Source: CAD feature listing. Evaluate the final solid. Frame: model axes, mm. A direction names the side the tool comes from. Give positions to 0.01 mm unless a question says otherwise; leave off trailing zeros. Loops run counter-clockwise (first coordinate to the right, second up) from the corner with the lowest first, then second, coordinate; pieces in that order, holes last. Notation, with made-up numbers: M 29,8.5 L 74,8.5 A27 cw 74,26.5 Z; hole C 74.25,73 d10. An arc over 180 degrees is marked long. Put each result on its own line as item: value.
from build123d import *

# Parameters (mm, degrees)
BOSS_EXTRUDE1_DEPTH = 5.18
CUT_EXTRUDE1_REACH  = 36.536
SKETCH2_W           = 3.45
SKETCH2_H           = 5.15
SKETCH3_W           = 10.5
SKETCH3_H           = 30
SKETCH3_R           = 1.575
BOSS_EXTRUDE2_DEPTH = 1.5
CUT_EXTRUDE3_REACH  = 43.242
SKETCH7_R           = 1.575


with BuildPart() as part:
    # Sketch1 → Boss-Extrude1 (new body)
    with BuildSketch(Plane(origin=(0, 0, 0), x_dir=(0, 0, -1), z_dir=(1, 0, 0))):
        Polygon((0, 0), (13, 0), (13, -7.5), (8.2, -7.5), (8.2, -11.6), (13.8, -11.6), (13.8, -10.716666667), (9.8, -10.716666667), (9.8, -10.9), (8.7, -10.9), (8.7, -8), (9.8, -8), (9.8, -8.183333333), (11.3, -8.183333333), (11.3, -8), (14.1, -8), (14.1, -8.183333333), (15.6, -8.183333333), (15.6, -8), (16.7, -8), (16.7, -9.1), (16.516666667, -9.1), (16.516666667, -11.1), (16.7, -11.1), (16.7, -16.35), (16.516666667, -16.35), (16.516666667, -18.35), (17.583333333, -18.35), (17.583333333, -16.35), (17.4, -16.35), (17.4, -11.1), (17.583333333, -11.1), (17.583333333, -9.1), (17.4, -9.1), (17.4, -8), (20.3, -8), (21.8, -19.95), (21.8, -21.45), (0, -21.45), (0, -24.78), (3, -24.78), (3, -26.28), (-1.5, -26.28), (-1.5, -19.95), (0, -8), (2.9, -8), (2.9, -9.5), (2.716666667, -9.5), (2.716666667, -11.5), (2.9, -11.5), (2.9, -16.15), (2.716666667, -16.15), (2.716666667, -18.15), (2.9, -18.15), (2.9, -18.333333333), (4.4, -18.333333333), (4.4, -18.15), (7.2, -18.15), (7.2, -18.333333333), (8.7, -18.333333333), (8.7, -17.266666667), (4.7, -17.266666667), (4.7, -17.45), (3.6, -17.45), (3.6, -7.5), (0, -7.5), align=None)
        Polygon((14.9, -9.8), (14.9, -15.65), (4.7, -15.65), (4.7, -16.533333333), (8.7, -16.533333333), (8.7, -16.35), (9.8, -16.35), (9.8, -19.25), (8.7, -19.25), (8.7, -19.066666667), (7.2, -19.066666667), (7.2, -19.25), (4.4, -19.25), (4.4, -19.066666667), (2.9, -19.066666667), (2.9, -19.25), (1.8, -19.25), (1.8, -18.15), (1.983333333, -18.15), (1.983333333, -16.15), (1.8, -16.15), (1.8, -11.5), (1.983333333, -11.5), (1.983333333, -9.5), (1.1, -9.5), (1.1, -19.95), (19.2, -19.95), (19.2, -9.1), (18.316666667, -9.1), (18.316666667, -11.1), (18.5, -11.1), (18.5, -16.35), (18.316666667, -16.35), (18.316666667, -18.35), (18.5, -18.35), (18.5, -19.45), (15.6, -19.45), (15.6, -18.35), (15.783333333, -18.35), (15.783333333, -16.35), (15.6, -16.35), (15.6, -11.1), (15.783333333, -11.1), (15.783333333, -9.1), (15.6, -9.1), (15.6, -8.916666667), (14.1, -8.916666667), (14.1, -9.1), (11.3, -9.1), (11.3, -8.916666667), (9.8, -8.916666667), (9.8, -9.983333333), (13.8, -9.983333333), (13.8, -9.8), align=None, mode=Mode.SUBTRACT)
    extrude(amount=BOSS_EXTRUDE1_DEPTH)

    # Sketch2 → Cut-Extrude1 (cut, up to next)
    with BuildSketch(Plane.XY, mode=Mode.PRIVATE) as cut_extrude1_sk1:
        with Locations((3.455, -3.425)):
            Rectangle(SKETCH2_W, SKETCH2_H)
    cut_extrude1_tool1 = extrude(cut_extrude1_sk1.sketch, amount=-CUT_EXTRUDE1_REACH, mode=Mode.PRIVATE) & part.part
    add(cut_extrude1_tool1.solids().sort_by_distance((3.455, -3.425, 0))[0], mode=Mode.SUBTRACT)

    # Sketch3 → Boss-Extrude2 (add)
    with BuildSketch(Plane.XZ.offset(21.45)):
        with Locations((5.25, -15)):
            Rectangle(SKETCH3_W, SKETCH3_H)
        with Locations(Location((7.62, -14.98, 0), (0, 0, 270))):
            Circle(SKETCH3_R, mode=Mode.SUBTRACT)
        with Locations(Location((7.62, -26.98, 0), (0, 0, 270))):
            Circle(SKETCH3_R, mode=Mode.SUBTRACT)
    extrude(amount=-BOSS_EXTRUDE2_DEPTH)

    # Sketch7 → Cut-Extrude3 (cut, up to next)
    with BuildSketch(Plane.ZY, mode=Mode.PRIVATE) as cut_extrude3_sk1:
        with Locations((-3.25, -3.5)):
            Circle(SKETCH7_R)
    cut_extrude3_tool1 = extrude(cut_extrude3_sk1.sketch, amount=-CUT_EXTRUDE3_REACH, mode=Mode.PRIVATE) & part.part
    # Sketch7 → Cut-Extrude3 (cut, up to next)
    with BuildSketch(Plane.ZY, mode=Mode.PRIVATE) as cut_extrude3_sk2:
        with Locations((-9.75, -3.5)):
            Circle(SKETCH7_R)
    cut_extrude3_tool2 = extrude(cut_extrude3_sk2.sketch, amount=-CUT_EXTRUDE3_REACH, mode=Mode.PRIVATE) & part.part
    add(cut_extrude3_tool1.solids().sort_by_distance((0, -3.5, -3.25))[0], mode=Mode.SUBTRACT)
    add(cut_extrude3_tool2.solids().sort_by_distance((0, -3.5, -9.75))[0], mode=Mode.SUBTRACT)


with BuildPart() as body_2:
    # Mirror3: mirrored copy
    add(part.part.mirror(Plane(origin=(0, 0, 0), x_dir=(0, 0, 1), z_dir=(1, 0, 0))))


solid = body_2.part
1. Section query B-B (x = -7.62). Output: boundary loops of the cut face in (y, z) (3 decimals), plus the area to 4 significant figures.
Found:
outline: M -21.45,-30 L -19.95,-30 L -19.95,-28.555 L -21.45,-28.555 Z; M -21.45,-25.405 L -19.95,-25.405 L -19.95,-16.555 L -21.45,-16.555 Z; M -21.45,-13.405 L -19.95,-13.405 L -19.95,0 L -21.45,0 Z
area: 35.55 mm^2
2. Access query for faces 4 (the flat face through (-3, -26.28, -1)), 5 (the flat face through (-3, -7.5, -2)), 6 (the flat face through (-3, -26, -3)), 7 (the flat face through (-3, -14, -18.5)). Directions: +Z, -Z, +X, -X, +Y, -Y. A direction counts if a zero-diameter tool reaches every point of the face in a straight line with its end or side. Return the directions, or none.
Found:
face 4: +Z, -Z, +X, -X, -Y
face 5: +Z, +X, -X
face 6: -Z, +X, -X, -Y
face 7: +X, -X
3. Material intervals for line 1 (Z direction, x = -7.62, y = -20.5) (3 decimals); line 2 (Y direction, x = -1.2, z = -3.25) (3 decimals); line 3 (Z direction, x = -2.75, y = -9.25), sorted ascending. Write a range as from..to.
Found:
line 1: -30..-28.555, -25.405..-16.555, -13.405..0
line 2: -21.45..-19.95, -19.067..-18.333, -7.5..-5.075, -1.925..0
line 3: -20.46..-19.2, -18.32..-17.58, -16.52..-15.78, -9.8..-8.7, -8.2..-3.6, -2.9..0.16
4. Section query A-A (y = -3.5). Output: boundary loops of the cut face in (x, z) (3 decimals), plus the area to 3 significant figures.
Found:
outline: M -1.73,-13 L 0,-13 L 0,-11.325 L -1.73,-11.325 Z; M -1.73,-8.175 L 0,-8.175 L 0,-4.825 L -1.73,-4.825 Z; M -1.73,-1.675 L 0,-1.675 L 0,0 L -1.73,0 Z
area: 11.6 mm^2
5. Section query D-D (y = -14). Output: boundary loops of the cut face in (x, z).
Found:
outline: M -5.18,-21.05 L 0,-21.05 L 0,-19.2 L -5.18,-19.2 Z; M -5.18,-18.5 L 0,-18.5 L 0,-17.4 L -5.18,-17.4 Z; M -5.18,-16.7 L 0,-16.7 L 0,-15.6 L -5.18,-15.6 Z; M -5.18,-14.9 L 0,-14.9 L 0,-3.6 L -5.18,-3.6 Z; M -5.18,-2.9 L 0,-2.9 L 0,-1.8 L -5.18,-1.8 Z; M -5.18,-1.1 L 0,-1.1 L 0,0.75 L -5.18,0.75 Z
6. Draft query along Y for faces 1 (the flat face through (-3, -17, -17.583)), 2 (the flat face through (-5, -21, -30)), 3 (the flat face through (-3, 0, -6)). Return one class per face: pulls with the +Y half, pulls with the -Y half, needs draft (parallel to the pull), parting line crosses it, or undercut.
Found:
face 1: undercut
face 2: needs draft
face 3: pulls with the +Y half
7. Contact query for flat-ended pins moving along their axis: P1, Ø1, axis at y = -22, z = -8.5, coming from the +X side; P2, Ø5.5, axis at x = -1.5, y = -14.5, coming from the +Z side; P3, Ø5.5, axis at x = -2.5, y = -3, coming from the +Z side; P4, Ø1, axis at x = -1.5, y = -17.5, coming from the -Z side. Output: stop coordinate, or through.
Found:
P1: through
P2: z = 1.16
P3: z = 0
P4: z = -21.56
8. Section query C-C (z = -4). Output: boundary loops of the cut face in (x, y).
Found:
outline: M -10.5,-21.45 L 0,-21.45 L 0,-19.95 L -10.5,-19.95 Z; M -5.18,-19.07 L 0,-19.07 L 0,-18.33 L -5.18,-18.33 Z; M -5.18,-17.45 L 0,-17.45 L 0,-4.88 L -1.73,-4.88 L -1.73,-6 L -5.18,-6 Z; M -5.18,-0.85 L -1.73,-0.85 L -1.73,-2.12 L 0,-2.12 L 0,0 L -5.18,0 Z
